Source: CAD feature listing. Evaluate the final solid. Frame: model axes, mm. Round coordinates to 2 decimals unless told otherwise and drop trailing zeros. Write each loop counter-clockwise with the first axis right and the second up, starting at its lowest first coordinate (ties: lowest second). Pieces come first, ordered by that corner, then holes.
from build123d import *

# Parameters (mm, degrees)
F1_DEPTH = 63.5
F2_R     = 5.08


with BuildPart() as f1:
    # F0 (on Top) → F1 (new body)
    with BuildSketch(Plane.XY):
        Polygon((0, 63.5), (0, 0), (63.5, 0), (63.5, 63.5), (31.75, 118.492613), align=None)
    extrude(amount=F1_DEPTH)

    # F2
    f2_edges = [f1.edges().sort_by_distance(p)[0] for p in [
        (15.875, 90.996307, 63.5),
        (0, 31.75, 63.5),
        (31.75, 0, 63.5),
        (63.5, 31.75, 63.5),
        (47.625, 90.996307, 63.5),
        (63.5, 0, 31.75),
        (63.5, 63.5, 31.75),
        (63.5, 31.75, 0),
        (31.75, 118.492613, 31.75),
        (47.625, 90.996307, 0),
        (0, 0, 31.75),
        (31.75, 0, 0),
        (0, 63.5, 31.75),
        (0, 31.75, 0),
        (15.875, 90.996307, 0),
    ]]
    fillet(f2_edges, radius=F2_R)


solid = f1.part
1) Section query A-A on z = 36.5. Return the cut outline in (x, y).
Taken from the geometry:
outline: (0, 5.08) arc R5.08 ccw to (5.08, 0) - (58.42, 0) arc R5.08 ccw to (63.5, 5.08) - (63.5, 62.14) arc R5.08 ccw to (62.82, 64.68) - (36.15, 110.87) arc R5.08 ccw to (27.35, 110.87) - (0.68, 64.68) arc R5.08 ccw to (0, 62.14) - close
2) Material intervals for line 1 (X direction, y = 69.5, z = 34); line 2 (X direction, y = 63, z = 60); line 3 (Y direction, x = 8.5, z = 25.5), sorted ascending.
Taken from the geometry:
line 1: x = 3.46 to 60.04
line 2: x = 0.33 to 63.17
line 3: y = 0 to 78.22
3) Contact query for flat-ended pins moving along their axis: P1, Ø3, axis at x = 28.5, y = 35, coming from the -Z side; P2, Ø1.5, axis at x = 36.5, z = 35, coming from the +Y side; P3, Ø4, axis at x = 13, z = 32.5, coming from the +Y side. Output: stop coordinate, or through.
Taken from the geometry:
P1: stops at z = 0
P2: stops at y = 111.46
P3: stops at y = 89.48
